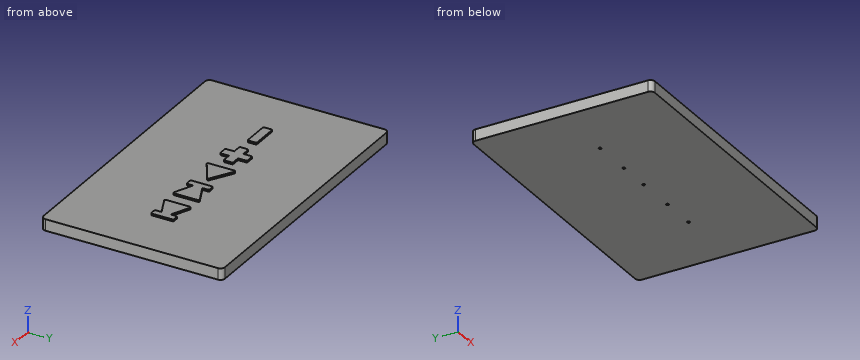
```python
from build123d import *

# Parameters (mm, degrees)
BOSS_EXTRUDE1_DEPTH = 5
BOSS_EXTRUDE2_DEPTH = 0.8
SKETCH22_R          = 0.6
CUT_EXTRUDE1_DEPTH  = 2


with BuildPart() as part:
    # Sketch1 → Boss-Extrude1 (new body)
    with BuildSketch(Plane.XY):
        with BuildLine():
            Line((-61, 40), (61, 40))
            ThreePointArc((61, 40), (62.414213562, 39.414213562), (63, 38))
            Line((63, 38), (63, -38))
            ThreePointArc((63, -38), (62.414213562, -39.414213562), (61, -40))
            Line((61, -40), (-61, -40))
            ThreePointArc((-61, -40), (-62.414213562, -39.414213562), (-63, -38))
            Line((-63, -38), (-63, 38))
            ThreePointArc((-63, 38), (-62.414213562, 39.414213562), (-61, 40))
        make_face()
    extrude(amount=BOSS_EXTRUDE1_DEPTH)

    # Sketch19 → Boss-Extrude2 (add)
    with BuildSketch(Plane.XY.offset(5)):
        with BuildLine():
            Line((-5, 5.7), (-5, -5.7))
            ThreePointArc((-5, -5.7), (-4.746349407, -6.135099953), (-4.242752122, -6.128746463))
            Line((-4.242752122, -6.128746463), (5.257247878, -0.428746463))
            ThreePointArc((5.257247878, -0.428746463), (5.5, 0), (5.257247878, 0.428746463))
            Line((5.257247878, 0.428746463), (-4.242752122, 6.128746463))
            ThreePointArc((-4.242752122, 6.128746463), (-4.746349407, 6.135099953), (-5, 5.7))
        make_face()
        with BuildLine():
            Line((-10, -1.5), (-10, 1.5))
            ThreePointArc((-10, 1.5), (-10.146446609, 1.853553391), (-10.5, 2))
            Line((-10.5, 2), (-14, 2))
            Line((-14, 2), (-14, 5.5))
            ThreePointArc((-14, 5.5), (-14.146446609, 5.853553391), (-14.5, 6))
            Line((-14.5, 6), (-17.5, 6))
            ThreePointArc((-17.5, 6), (-17.853553391, 5.853553391), (-18, 5.5))
            Line((-18, 5.5), (-18, 2))
            Line((-18, 2), (-21.5, 2))
            ThreePointArc((-21.5, 2), (-21.853553391, 1.853553391), (-22, 1.5))
            Line((-22, 1.5), (-22, -1.5))
            ThreePointArc((-22, -1.5), (-21.853553391, -1.853553391), (-21.5, -2))
            Line((-21.5, -2), (-18, -2))
            Line((-18, -2), (-18, -5.5))
            ThreePointArc((-18, -5.5), (-17.853553391, -5.853553391), (-17.5, -6))
            Line((-17.5, -6), (-14.5, -6))
            ThreePointArc((-14.5, -6), (-14.146446609, -5.853553391), (-14, -5.5))
            Line((-14, -5.5), (-14, -2))
            Line((-14, -2), (-10.5, -2))
            ThreePointArc((-10.5, -2), (-10.146446609, -1.853553391), (-10, -1.5))
        make_face()
        with BuildLine():
            Line((-28, 1.5), (-28, -1.5))
            ThreePointArc((-28, -1.5), (-28.146446609, -1.853553391), (-28.5, -2))
            Line((-28.5, -2), (-39.5, -2))
            ThreePointArc((-39.5, -2), (-39.853553391, -1.853553391), (-40, -1.5))
            Line((-40, -1.5), (-40, 1.5))
            ThreePointArc((-40, 1.5), (-39.853553391, 1.853553391), (-39.5, 2))
            Line((-39.5, 2), (-28.5, 2))
            ThreePointArc((-28.5, 2), (-28.146446609, 1.853553391), (-28, 1.5))
        make_face()
        with BuildLine():
            Line((10, 4.5), (10, -4.5))
            ThreePointArc((10, -4.5), (10.146446609, -4.853553391), (10.5, -5))
            Line((10.5, -5), (12.5, -5))
            ThreePointArc((12.5, -5), (12.853553391, -4.853553391), (13, -4.5))
            Line((13, -4.5), (13, -2))
            Line((13, -2), (21.296930767, -5.687524785))
            ThreePointArc((21.296930767, -5.687524785), (21.77245677, -5.64986513), (22, -5.230619011))
            Line((22, -5.230619011), (22, 5.230619011))
            ThreePointArc((22, 5.230619011), (21.77245677, 5.64986513), (21.296930767, 5.687524785))
            Line((21.296930767, 5.687524785), (13, 2))
            Line((13, 2), (13, 4.5))
            ThreePointArc((13, 4.5), (12.853553391, 4.853553391), (12.5, 5))
            Line((12.5, 5), (10.5, 5))
            ThreePointArc((10.5, 5), (10.146446609, 4.853553391), (10, 4.5))
        make_face()
        with BuildLine():
            Line((28, 5.230619011), (28, -5.230619011))
            ThreePointArc((28, -5.230619011), (28.22754323, -5.64986513), (28.703069233, -5.687524785))
            Line((28.703069233, -5.687524785), (37, -2))
            Line((37, -2), (37, -4.5))
            ThreePointArc((37, -4.5), (37.146446609, -4.853553391), (37.5, -5))
            Line((37.5, -5), (39.5, -5))
            ThreePointArc((39.5, -5), (39.853553391, -4.853553391), (40, -4.5))
            Line((40, -4.5), (40, 4.5))
            ThreePointArc((40, 4.5), (39.853553391, 4.853553391), (39.5, 5))
            Line((39.5, 5), (37.5, 5))
            ThreePointArc((37.5, 5), (37.146446609, 4.853553391), (37, 4.5))
            Line((37, 4.5), (37, 2))
            Line((37, 2), (28.703069233, 5.687524785))
            ThreePointArc((28.703069233, 5.687524785), (28.22754323, 5.64986513), (28, 5.230619011))
        make_face()
    extrude(amount=BOSS_EXTRUDE2_DEPTH)

    # Sketch22 → Cut-Extrude1 (cut)
    with BuildSketch(Plane.XY):
        with Locations((-34, 0)):
            Circle(SKETCH22_R)
        with Locations((-16, 0)):
            Circle(SKETCH22_R)
        with Locations((-1, 0)):
            Circle(SKETCH22_R)
        with Locations((17, 0)):
            Circle(SKETCH22_R)
        with Locations((33, 0)):
            Circle(SKETCH22_R)
    extrude(amount=CUT_EXTRUDE1_DEPTH, mode=Mode.SUBTRACT)


solid = part.part
```
Verification items for the finished model (mm, model axes). Round coordinates to 2 decimals unless told otherwise and drop trailing zeros. Order: outer loops, then holes, each group sorted by start corner. A loop starts at its lowest first (then second) coordinate and runs counter-clockwise, first axis right, second up. Notation, with made-up numbers: (79.5, 41.5) - (99.5, 41.5) arc R26 cw to (99.5, 74.5) - close; hole circle Ø9 at (87.5, -15). An arc over 180 degrees is marked (long way). Use CSV: the item, a comma, the result in double quotes. Start each with the question number.
1) Go/stop test with flat-tipped pins: P1, Ø0.9, axis at y = -2.5, z = 5.5, coming from the -X side; P2, Ø0.6, axis at y = 0.5, z = 5.5, coming from the -X side; P3, Ø2, axis at x = 11, y = 7.5, coming from the -Z side; P4, Ø8, axis at x = 22.5, y = -22.5, coming from the +Z side. Record where each tip stops, or that it passes through.
2) Section check A-A, the plane x = -55. Record the cut outline in (y, z), plus the area to 3 significant figures.
3) Thickness scan on L1, parallel to Y at x = -1, z = 0.8; L2, parallel to Z at x = 34.5, y = 22. Record the ranges inside material, lowest first.
4) Section check B-B, the plane y = 22. Record the cut outline in (x, z), plus the area to 3 significant figures.
Answers:
1,P1,"stops at x = -18"
1,P2,"stops at x = -40"
1,P3,"stops at z = 0"
1,P4,"stops at z = 5"
2,outline,"(-40, 0) - (40, 0) - (40, 5) - (-40, 5) - close"
2,area,"400 mm²"
3,L1,"y = -40 to -0.6, 0.6 to 40"
3,L2,"z = 0 to 5"
4,outline,"(-63, 0) - (63, 0) - (63, 5) - (-63, 5) - close"
4,area,"630 mm²"
